```python
from build123d import *

# Parameters (mm, degrees)
F1_DEPTH = 25.4


with BuildPart() as f1:
    # F0 (on Front) → F1 (new body, symmetric)
    with BuildSketch(Plane.XZ):
        Polygon((-41.275, -9.525), (41.275, -9.525), (41.275, 9.525), (22.225, 9.525), (-41.275, 9.525), align=None)
        with BuildLine():
            Line((22.225, 9.525), (41.275, 9.525))
            Line((41.275, 9.525), (41.275, 27.0002))
            ThreePointArc((41.275, 27.0002), (45.92468, 38.22552), (57.15, 42.8752))
            Line((57.15, 42.8752), (73.025, 42.8752))
            Line((73.025, 42.8752), (73.025, 43.09893))
            Line((73.025, 43.09893), (73.025, 61.9252))
            Line((73.025, 61.9252), (57.15, 61.9252))
            ThreePointArc((57.15, 61.9252), (32.454296, 51.695904), (22.225, 27.0002))
            Line((22.225, 27.0002), (22.225, 9.525))
        make_face()
        Polygon((73.025, 43.09893), (73.025, 42.8752), (73.025, 38.1), (98.425, 38.1), (98.425, 66.675), (73.025, 66.675), (73.025, 61.9252), align=None)
    extrude(amount=F1_DEPTH, both=True)


solid = f1.part
```
Work out the finished part from the listing and answer in its coordinate system (mm). A direction names the side the tool comes from. Round coordinates to 2 decimals unless told otherwise and drop trailing zeros. Write each loop counter-clockwise with the first axis right and the second up, starting at its lowest first coordinate (ties: lowest second). Pieces come first, ordered by that corner, then holes. Notation, with made-up numbers: (74.25, -36.75) - (116.25, -36.75) arc R23 cw to (116.25, -0.75) - close; hole circle Ø8 at (-29.75, -2). An arc over 180 degrees is marked (long way). Return JSON: item names as keys, results as strings. Group by question number.
Q1. Each of these flat-tipped pins is pushed along its axis until it touches: pin 1 Ø8 at (x, y) = (68, 5.5) entering from +Z; pin 2 Ø10 at (y, z) = (0, 20.5) entering from -X (3 decimals); pin 3 Ø1.4 at (y, z) = (6.5, 64) entering from -X (3 decimals). Where does it stop, or does it pass through?
Q2. The part is cut by section B-B on x = 87.5. Write down the section's boundary in (y, z) (3 decimals).
Q3. For faces 1 (the flat face through (41.275, 0, 8)), 2 (the flat face through (-9, 0, 9.525)), 3 (the flat face through (65, 0, 42.875)), 4 (the flat face through (98.425, 0, 52)), 5 (the flat face through (-41.275, 0, 0)), determine the directions among +Z, -Z, +X, -X, +Y, -Y from which every point of the face is accessible in a straight line to the end or side of a thin tool.
Q4. The part is cut by section A-A on y = 8. Write down the section's boundary in (x, z) (3 decimals).
Q5. Find the intervals of material crossed by L1, parallel to X at y = 0, z = 5.5 (3 decimals); L2, parallel to Z at x = 78, y = -13.5 (3 decimals); L3, parallel to Z at x = 64.5, y = 5, in increasing order.
Q6. The mould has two halves that part along X. Classify faces 6 (the flat face through (-1, 0, -9.525)), 7 (the cylindrical face through (45.8, -0.4, 38.1)), 8 (the flat face through (73.025, 0, 64)), 9 (the flat face through (73.025, 0, 41)): released by +X, released by -X, zero draft, split by the parting line, or undercut.
Q7. The part is cut by section C-C on z = 7. Write down the section's boundary in (x, y) (3 decimals), then the cut area to 3 significant figures.
Solved:
{
 "1": {"pin 1": "z = 61.93", "pin 2": "x = 22.225", "pin 3": "x = 73.025"},
 "2": {"outline": "(-25.4, 38.1) - (25.4, 38.1) - (25.4, 66.675) - (-25.4, 66.675) - close"},
 "3": {"face 1": "-Z, +X, +Y, -Y", "face 2": "+Z, -X, +Y, -Y", "face 3": "-Z, +Y, -Y", "face 4": "+Z, -Z, +X, +Y, -Y", "face 5": "+Z, -Z, -X, +Y, -Y"},
 "4": {"outline": "(-41.275, -9.525) - (41.275, -9.525) - (41.275, 27) arc R15.875 cw to (57.15, 42.875) - (73.025, 42.875) - (73.025, 38.1) - (98.425, 38.1) - (98.425, 66.675) - (73.025, 66.675) - (73.025, 61.925) - (57.15, 61.925) arc R34.925 ccw to (22.225, 27) - (22.225, 9.525) - (-41.275, 9.525) - close"},
 "5": {"L1": "-41.275 to 41.275", "L2": "38.1 to 66.675", "L3": "42.88 to 61.93"},
 "6": {"face 6": "zero draft", "face 7": "undercut", "face 8": "released by -X", "face 9": "undercut"},
 "7": {"outline": "(-41.275, -25.4) - (41.275, -25.4) - (41.275, 25.4) - (-41.275, 25.4) - close", "area": "4,190 mm²"}
}
